from build123d import *

# Parameters (mm, degrees)
F0_R     = 25.4
F0_R_2   = 2.3876
F1_DEPTH = 25.4
F2_R     = 15.875
F3_DEPTH = 12.7
F4_R     = 15.875
F4_R_2   = 6.35
F5_DEPTH = 6.35
F6_R     = 2.3876
F7_DEPTH = 12.701


with BuildPart() as f1:
    # F0 (on Top) → F1 (new body)
    with BuildSketch(Plane.XY):
        Circle(F0_R)
        Circle(F0_R_2, mode=Mode.SUBTRACT)
    extrude(amount=F1_DEPTH)

    # F2 (on face) → F3 (cut)
    with BuildSketch(Plane.XY.offset(25.4)):
        Circle(F2_R)
    extrude(amount=-F3_DEPTH, mode=Mode.SUBTRACT)

    # F4 (on face) → F5 (cut)
    with BuildSketch(Plane(origin=(0, 0, 0), x_dir=(1, 0, 0), z_dir=(0, 0, -1))):
        Circle(F4_R)
        Circle(F4_R_2, mode=Mode.SUBTRACT)
    extrude(amount=-F5_DEPTH, mode=Mode.SUBTRACT)

    # F6 (on face) → F7 (cut, through all)
    with BuildSketch(Plane.XY.offset(12.7)):
        with BuildLine():
            ThreePointArc((7.6596854017, 8.0508928571), (6.8740766425, 3.96875), (10.8021204383, 2.6080357143))
            ThreePointArc((10.8021204383, 2.6080357143), (9.6237072996, 5.55625), (7.6596854017, 8.0508928571))
        make_face()
        with BuildLine():
            ThreePointArc((7.6596854017, 8.0508928571), (9.6237072996, 5.55625), (10.8021204383, 2.6080357143))
            ThreePointArc((10.8021204383, 2.6080357143), (12.2525936337, 3.775918109), (12.7987072996, 5.55625))
            ThreePointArc((12.7987072996, 5.55625), (11.010223703, 8.4125058119), (7.6596854017, 8.0508928571))
        make_face()
        with BuildLine():
            ThreePointArc((12.7987072996, -5.55625), (12.2525936337, -3.775918109), (10.8021204383, -2.6080357143))
            ThreePointArc((10.8021204383, -2.6080357143), (9.6237072996, -5.55625), (7.6596854017, -8.0508928571))
            ThreePointArc((7.6596854017, -8.0508928571), (11.010223703, -8.4125058119), (12.7987072996, -5.55625))
        make_face()
        with BuildLine():
            ThreePointArc((7.6596854017, -8.0508928571), (9.6237072996, -5.55625), (10.8021204383, -2.6080357143))
            ThreePointArc((10.8021204383, -2.6080357143), (6.8740766425, -3.96875), (7.6596854017, -8.0508928571))
        make_face()
        with BuildLine():
            ThreePointArc((-3.1424350366, 10.6589285714), (0, 7.9375), (3.1424350366, 10.6589285714))
            ThreePointArc((3.1424350366, 10.6589285714), (0, 11.1125), (-3.1424350366, 10.6589285714))
        make_face()
        with BuildLine():
            ThreePointArc((-3.1424350366, 10.6589285714), (0, 11.1125), (3.1424350366, 10.6589285714))
            ThreePointArc((3.1424350366, 10.6589285714), (3.1668482945, 10.8851305222), (3.175, 11.1125))
            ThreePointArc((3.175, 11.1125), (-0.2273694778, 14.2793482945), (-3.1424350366, 10.6589285714))
        make_face()
        with BuildLine():
            ThreePointArc((3.175, -11.1125), (3.1668482945, -10.8851305222), (3.1424350366, -10.6589285714))
            ThreePointArc((3.1424350366, -10.6589285714), (0, -11.1125), (-3.1424350366, -10.6589285714))
            ThreePointArc((-3.1424350366, -10.6589285714), (-0.2273694778, -14.2793482945), (3.175, -11.1125))
        make_face()
        with BuildLine():
            ThreePointArc((-3.1424350366, -10.6589285714), (0, -11.1125), (3.1424350366, -10.6589285714))
            ThreePointArc((3.1424350366, -10.6589285714), (0, -7.9375), (-3.1424350366, -10.6589285714))
        make_face()
        with BuildLine():
            ThreePointArc((-6.4487072996, 5.55625), (-6.7674514877, 6.9427664035), (-7.6596854017, 8.0508928571))
            ThreePointArc((-7.6596854017, 8.0508928571), (-9.6237072996, 5.55625), (-10.8021204383, 2.6080357143))
            ThreePointArc((-10.8021204383, 2.6080357143), (-7.8433754085, 2.9273636659), (-6.4487072996, 5.55625))
        make_face()
        with BuildLine():
            ThreePointArc((-10.8021204383, 2.6080357143), (-9.6237072996, 5.55625), (-7.6596854017, 8.0508928571))
            ThreePointArc((-7.6596854017, 8.0508928571), (-12.3733379566, 7.14375), (-10.8021204383, 2.6080357143))
        make_face()
        with BuildLine():
            ThreePointArc((-10.8021204383, -2.6080357143), (-12.3733379566, -7.14375), (-7.6596854017, -8.0508928571))
            ThreePointArc((-7.6596854017, -8.0508928571), (-9.6237072996, -5.55625), (-10.8021204383, -2.6080357143))
        make_face()
        with BuildLine():
            ThreePointArc((-10.8021204383, -2.6080357143), (-9.6237072996, -5.55625), (-7.6596854017, -8.0508928571))
            ThreePointArc((-7.6596854017, -8.0508928571), (-6.7674514877, -6.9427664035), (-6.4487072996, -5.55625))
            ThreePointArc((-6.4487072996, -5.55625), (-7.8433754085, -2.9273636659), (-10.8021204383, -2.6080357143))
        make_face()
        Circle(F6_R)
    extrude(amount=-F7_DEPTH, mode=Mode.SUBTRACT)


solid = f1.part
CAD build for the part. Positions are in the model's coordinates, mm. A direction names the side the tool comes from. Give positions to 0.01 mm unless a question says otherwise; leave off trailing zeros. Order: outer loops, then holes, each group sorted by start corner. A loop starts at its lowest first (then second) coordinate and runs counter-clockwise, first axis right, second up. Notation, with made-up numbers: (51.5, 5) - (110.5, 5) arc R29 cw to (110.5, 37) - close; hole circle Ø2 at (-40, -14). An arc over 180 degrees is marked (long way). Answer in a Markdown table with one row per item.
1. Saw through at A-A, the plane y = 0. Give the cut face in (x, z) (3 decimals).
Data:
| item | result |
|---|---|
| outline | (-25.4, 0) - (-15.875, 0) - (-15.875, 6.35) - (-6.35, 6.35) - (-6.35, 0) - (-2.388, 0) - (-2.388, 12.7) - (-15.875, 12.7) - (-15.875, 25.4) - (-25.4, 25.4) - close; (2.388, 0) - (6.35, 0) - (6.35, 6.35) - (15.875, 6.35) - (15.875, 0) - (25.4, 0) - (25.4, 25.4) - (15.875, 25.4) - (15.875, 12.7) - (2.388, 12.7) - close |
2. Saw through at D-D, the plane x = 9.5. Give the cut face in (y, z), plus the area to 3 significant figures.
Data:
| item | result |
|---|---|
| outline | (-23.56, 0) - (-12.72, 0) - (-12.72, 6.35) - (-8.73, 6.35) - (-8.73, 12.7) - (-12.72, 12.7) - (-12.72, 25.4) - (-23.56, 25.4) - close; (-2.38, 6.35) - (2.38, 6.35) - (2.38, 12.7) - (-2.38, 12.7) - close; (8.73, 6.35) - (12.72, 6.35) - (12.72, 0) - (23.56, 0) - (23.56, 25.4) - (12.72, 25.4) - (12.72, 12.7) - (8.73, 12.7) - close |
| area | 632 mm² |
3. Saw through at B-B, the plane x = 0. Count the separate pieces of the cut face and the enclosed holes in it, plus the area to 3 significant figures.
Data:
| item | result |
|---|---|
| separate pieces | 4 |
| enclosed holes | 0 |
| area | 625 mm² |
4. Flat gauge pins, fed straight in: pin 1 (16 mm diameter, centred on x = 4.5, y = -5.5, fed in from +Z); pin 2 (8 mm diameter, centred on y = -5.5, z = 6.5, fed in from +X); pin 3 (4 mm diameter, centred on x = 0, y = 0, fed in from +Z); pin 4 (8 mm diameter, centred on y = -9.5, z = 22, fed in from -X). Where does each tip first touch, or does it go through?
Data:
| item | result |
|---|---|
| pin 1 | stops at z = 12.7 |
| pin 2 | stops at x = 25.36 |
| pin 3 | passes through |
| pin 4 | stops at x = -24.8 |
5. Pull direction Y, two halves, no side cores. Call faces 1 (the cylindrical face through (-5.506, -24.796, 12.522)), 2 (the flat face through (7, 0, 6.35)), 3 (the flat face through (11, 12, 25.4)): pulls with the +Y half, pulls with the -Y half, needs draft (parallel to the pull), parting line crosses it, or undercut.
Data:
| item | result |
|---|---|
| face 1 | parting line crosses it |
| face 2 | undercut |
| face 3 | needs draft |
6. Tool access for faces 4 (the cylindrical face through (-3.441, -15.497, 19.139)), 5 (the cylindrical face through (-0.52, -2.33, 6.26)), 6 (the cylindrical face through (-3.441, 15.497, 3.131)): list every direction of +Z, -Z, +X, -X, +Y, -Y with a clear straight run to the whole face (end or side of a thin tool).
Data:
| item | result |
|---|---|
| face 4 | +Z |
| face 5 | +Z, -Z |
| face 6 | -Z |
7. Probe probe 1 along Y at (x, z) = (0, 3.25) (3 decimals); probe 2 along Y at (x, z) = (0, 21.75) (3 decimals); probe 3 along Y at (x, z) = (9.5, 7.75). List the from-to ranges inside material, lowest first. Write a range as [from, to].
Data:
| item | result |
|---|---|
| probe 1 | y = [-25.4, -15.875], [-6.35, -2.388], [2.388, 6.35], [15.875, 25.4] |
| probe 2 | y = [-25.4, -15.875], [15.875, 25.4] |
| probe 3 | y = [-23.56, -8.73], [-2.38, 2.38], [8.73, 23.56] |
